The model under review builds one solid part; all positions refer to its coordinate system, in mm. Coordinates: 2 decimals unless noted, no trailing zeros. Write each loop counter-clockwise with the first axis right and the second up, starting at its lowest first coordinate (ties: lowest second). Pieces come first, ordered by that corner, then holes. Notation, with made-up numbers: (32, 2.5) - (61, 2.5) arc R18 cw to (61, 20.5) - close; hole circle Ø2 at (-38.5, -7.5). An arc over 180 degrees is marked (long way). Use one line per item in the form item = value. Start each with the question number.
Autodesk Inventor part; units mm, degrees
ref_plane "YZ Plane" through (0, 0, 0) normal (1, 0, 0) x (0, 1, 0)
ref_plane "XZ Plane" through (0, 0, 0) normal (0, 1, 0) x (-1, 0, 0)
ref_plane "XY Plane" through (0, 0, 0) normal (0, 0, 1) x (1, 0, 0)
sketch "Sketch1" plane through (0, 0, 0) normal (0, 1, 0) x (-1, 0, 0)
  line L0 (-22.225, 22.225) -> (-22.225, -22.225)
  line L1 (-22.225, -22.225) -> (22.225, -22.225)
  line L2 (22.225, -22.225) -> (22.225, 22.225)
  line L3 (22.225, 22.225) -> (-22.225, 22.225)
  line L4 (-22.225, 22.225) -> (22.225, -22.225) construction
  line L5 (-22.225, -22.225) -> (22.225, 22.225) construction
  point P0 (0, 0)
  dimension "d4" = 44.45
extrude "Extrusion1" add sketch "Sketch1" along normal blind 25.4
sketch "Sketch3" plane through (-22.225, 0, 22.225) normal (0, 0, 1) x (1, 0, 0)
  line L0 (44.45, 25.4) -> (0, 25.4) construction
  point P0 (22.225, 0)
  point P1 (22.225, 25.4)
  point P2 (22.225, 0)
hole "Hole1" at (0, 25.4, 22.225) at (0, 0, 22.225) direction (0, 0, -1) diameter 9.525 end through all
sketch "Sketch4" plane through (0, 25.4, 0) normal (0, 1, 0) x (1, 0, 0)
  line L0 (-22.225, 22.225) -> (-22.225, -22.225)
  line L1 (22.225, -22.225) -> (22.225, 22.225)
  line L2 (-22.225, -22.225) -> (-4.7625, -22.225)
  line L3 (4.7625, -22.225) -> (22.225, -22.225)
  point P0 (0, 0)
  point P1 (-13.4938, 0)
  point P2 (13.4938, 0)
  dimension "d16" = 8.7312
  dimension "d17" = 8.7312
  dimension "d25" = 22.225
  dimension "d26" = 22.225
hole "Hole2" at (-13.4938, 25.4, 0) at (13.4938, 25.4, 0) direction (0, -1, 0) diameter 5.1054 end through all
sketch "Sketch5" plane through (0, 25.4, 0) normal (0, 1, 0) x (1, 0, 0)
  line L0 (-13.4938, -13.4938) -> (13.4938, -13.4938) construction
  line L1 (13.4938, -13.4938) -> (13.4938, 13.4938) construction
  line L2 (13.4938, 13.4938) -> (-13.4938, 13.4938) construction
  line L3 (-13.4938, 13.4938) -> (-13.4938, -13.4938) construction
  line L4 (-13.4938, -13.4938) -> (13.4938, 13.4938) construction
  line L5 (13.4938, -13.4938) -> (-13.4938, 13.4938) construction
  line L6 (-22.225, -22.225) -> (-4.7625, -22.225)
  line L7 (-22.225, 22.225) -> (-22.225, -22.225)
  circle A0 centre (-13.4938, -13.4938) radius 2.794
  circle A1 centre (13.4938, -13.4938) radius 2.794
  circle A2 centre (13.4938, 13.4938) radius 2.794
  circle A3 centre (-13.4938, 13.4938) radius 2.794
  point P0 (0, 0)
  dimension "d27" = 8.7312
  dimension "d28" = 8.7312
  dimension "d29" = 5.588
extrude "Extrusion2" cut sketch "Sketch5" against normal through all
equation "\"d4\" = baseWidth"
equation "\"d6\" = heightOfMiddleSection"
equation "\"d9\" = bottomHoleDiam"
equation "\"d27\" = edgeToBoltHole"
equation "\"d28\" = edgeToBoltHole"
equation "\"d29\" = supportHoleDiam"
equation "\"bottomHoleDiam\" = 9.525"
equation "\"baseWidth\" = 44.45"
equation "\"deltaBottomToTop\" = 27.94"
equation "\"d0\" = baseWidth"
equation "\"d1\" = heightOfBottomHole"
equation "\"d2\" = 0"
equation "\"d3\" = bottomHoleDiam"
equation "\"d5\" = 0"
equation "\"height\" = deltaBottomToTop + heightOfBottomHole + heightOfTopHole"
equation "\"topHoleDiam\" = 9.525"
equation "\"edgeToBoltHole\" = -0.25 * bottomHoleDiam + 0.25 * baseWidth"
equation "\"heightOfMiddleSection\" = 25.4"
equation "\"baseLength\" = 44.45"
equation "\"supportHoleDiam\" = 5.588"
properties part number "MiddleOfSquareSupport" material "PC/ABS Plastic"
1. The part is to be moulded in two halves that separate along Z. For faces 1 (the flat face through (0, 13, -22.225)), 2 (the flat face through (22.225, 13, 0)), 3 (the cylindrical face through (14.783, 12.878, -11.015)), say which applies: released by +Z, released by -Z, zero draft, split by the parting line, or undercut.
2. For L1, parallel to X at y = 17.75, z = 0 (1 decimal); L2, parallel to Z at x = 13.5, y = 10.5 (3 decimals); L3, parallel to X at y = 14.5, z = -14.5 (3 decimals), list the stretches that pass through material, from the lowest coordinate up.
3. Take a section at B-B (y = 23). State the section outline as (x, z) points (3 decimals).
4. Take a section at C-C (z = -18). State the section outline as (x, y) points (1 decimal).
5. For P1, Ø6.5, axis at x = 13.49, z = 13.49, coming from the +Y side; P2, Ø5, axis at x = -1, z = -9, coming from the +Y side, all flat-tipped, find the tip position at first contact; note any pin that passes through.
6. Take a section at D-D (y = 15). State the section outline as (x, z) points (3 decimals).
7. Take a section at A-A (z = 0). State the section outline as (x, y) points (1 decimal).
Returned:
q1.face_1 = released by -Z
q1.face_2 = zero draft
q1.face_3 = undercut
q2.L1 = -22.2 to -16, -10.9 to 10.9, 16 to 22.2
q2.L2 = -22.225 to -16.288, -10.7 to -2.553, 2.553 to 10.7, 16.288 to 22.225
q2.L3 = -22.225 to -16.1, -10.887 to 10.887, 16.1 to 22.225
q3.outline = (-22.225, -22.225) - (-4.114, -22.225) - (-4.114, 22.225) - (-22.225, 22.225) - close; (4.114, -22.225) - (22.225, -22.225) - (22.225, 22.225) - (4.114, 22.225) - close; hole circle Ø5.588 at (-13.494, -13.494); hole circle Ø5.588 at (-13.494, 13.494); hole circle Ø5.105 at (-13.494, 0); hole circle Ø5.588 at (13.494, -13.494); hole circle Ø5.588 at (13.494, 13.494); hole circle Ø5.105 at (13.494, 0)
q4.outline = (-22.2, 0) - (-4.8, 0) arc R4.8 cw to (4.8, 0) - (22.2, 0) - (22.2, 25.4) - (4.8, 25.4) arc R4.8 cw to (-4.8, 25.4) - (-22.2, 25.4) - close
q5.P1 = 25.4
q5.P2 = 22.17
q6.outline = (-22.225, -22.225) - (22.225, -22.225) - (22.225, 22.225) - (-22.225, 22.225) - close; hole circle Ø5.588 at (-13.494, -13.494); hole circle Ø5.588 at (-13.494, 13.494); hole circle Ø5.105 at (-13.494, 0); hole circle Ø5.588 at (13.494, -13.494); hole circle Ø5.588 at (13.494, 13.494); hole circle Ø5.105 at (13.494, 0)
q7.outline = (-22.2, 0) - (-16, 0) - (-16, 25.4) - (-22.2, 25.4) - close; (-10.9, 0) - (-4.8, 0) arc R4.8 cw to (4.8, 0) - (10.9, 0) - (10.9, 25.4) - (4.8, 25.4) arc R4.8 cw to (-4.8, 25.4) - (-10.9, 25.4) - close; (16, 0) - (22.2, 0) - (22.2, 25.4) - (16, 25.4) - close
